Source: CAD feature listing. Evaluate the final solid. Frame: model axes, mm. Face numbers are marked on the shaded views. A direction names the side the tool comes from. Round coordinates to 2 decimals unless told otherwise and drop trailing zeros. Order: outer loops, then holes, each group sorted by start corner. A loop starts at its lowest first (then second) coordinate and runs counter-clockwise, first axis right, second up. Notation, with made-up numbers: (64.5, 28) - (84.5, 28) arc R20 ccw to (84.5, 32) - close; hole circle Ø11 at (18, 68.5). An arc over 180 degrees is marked (long way). Return JSON: item names as keys, results as strings. Group by question number.
1) Contact query for flat-ended pins moving along their axis: P1, Ø4, axis at y = -20, z = 15.5, coming from the -X side; P2, Ø4, axis at x = -21.5, y = -4.5, coming from the -Z side; P3, Ø3, axis at x = -20.5, y = -11.5, coming from the +Z side; P4, Ø10, axis at y = -18.5, z = -10, coming from the +X side. Output: stop coordinate, or through.
2) Section D-D, the plane y = -6.5. Return loops of the section in (x, z), plus the area to 3 significant figures.
3) Ray query, line 1 (X direction, y = -15.75, z = 2); line 2 (X direction, y = -6.75, z = -2); line 3 (Z direction, x = 13.5, y = -12.5). Return the intervals inside material, ascending. Write a range as from..to.
4) Section B-B, the plane x = 23.5. Return loops of the section in (y, z).
5) Access query for the marked faces 1, 2 and 3. Directions: +Z, -Z, +X, -X, +Y, -Y. A direction counts if a zero-diameter tool reaches every point of the face in a straight line with its end or side. Return the directions, or none.
6) Mould query, pull axis Z, two halves, no side actions, for the marked faces 4, 5, 6 and 7. Classes: pulls with the +Z half, pulls with the -Z half, needs draft (parallel to the pull), parting line crosses it, or undercut.
7) Section C-C, the plane y = -16.5. Return loops of the section in (x, z).
8) Section A-A, the plane z = -23.5. Return loops of the section in (x, y), plus the area to 3 significant figures.
```python
from build123d import *

# Parameters (mm, degrees)
F1_DEPTH = 25.4
F2_R     = 8.4230292531
F3_DEPTH = 15.24
F4_R     = 8.4646694798
F5_DEPTH = 15.24


with BuildPart() as f1:
    # F0 (on Front) → F1 (new body)
    with BuildSketch(Plane.XZ):
        Polygon((0, 51.8097877502), (-6.8899182792, 21.4846514834), (-38.7902185321, 21.4846514834), (-14.4291445613, 0), (-23.4517641366, -28.4915324301), (0, -12.2508164495), (27.0749107003, -28.4915324301), (18.9545508474, 0), (43.3156266809, 21.4846514834), (12.6387169585, 21.4846514834), align=None)
    extrude(amount=F1_DEPTH)

    # F2 (on face) → F3 (cut)
    with BuildSketch(Plane(origin=(-5.4041094275, 0, -9.0091951821), x_dir=(0.8575520342, 0, -0.5143972285), z_dir=(-0.5143972285, 0, -0.8575520342))):
        with Locations((6.3017860283, 12.7)):
            Circle(F2_R)
    extrude(amount=-F3_DEPTH, mode=Mode.SUBTRACT)

    # F4 (on face) → F5 (cut)
    with BuildSketch(Plane(origin=(5.7339883167, 0, -8.279939242), x_dir=(0.8221121344, 0, 0.5693255996), z_dir=(0.5693255996, 0, -0.8221121344))):
        with Locations((-6.9747034212, 12.7)):
            Circle(F4_R)
    extrude(amount=-F5_DEPTH, mode=Mode.SUBTRACT)


solid = f1.part
```
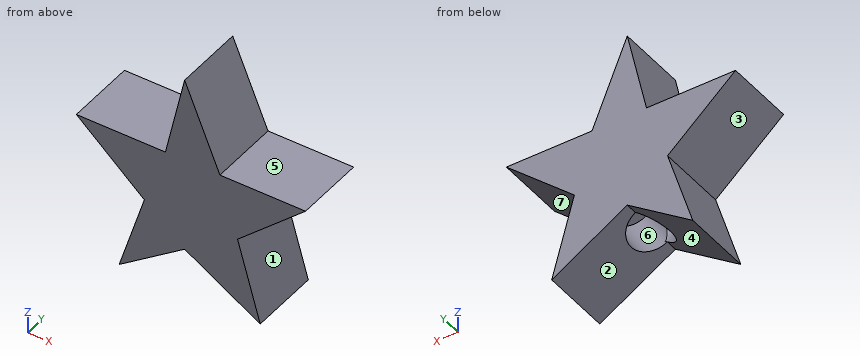
Geometry check:
{
 "1": {"P1": "x = -34.27", "P2": "z = -28.49", "P3": "z = 21.48", "P4": "x = 23.23"},
 "2": {"outline": "(-38.79, 21.48) - (-14.43, 0) - (-23.45, -28.49) - (-4.74, -15.53) - (-13.41, -3) - (-3.94, 3.56) - (-0.31, -1.68) - (2.95, 3.75) - (12.73, -2.11) - (4.89, -15.18) - (27.07, -28.49) - (18.95, 0) - (43.32, 21.48) - (12.64, 21.48) - (0, 51.81) - (-6.89, 21.48) - close", "area": "2,020 mm2"},
 "3": {"line 1": "-16.7..-6.19, 5.87..21.22", "line 2": "-15.06..-11.97, 12.54..19.52", "line 3": "-20.35..-6.11, -2.58..21.48"},
 "4": {"outline": "(-25.4, -26.35) - (0, -26.35) - (0, -15.95) - (-25.4, -15.95) - close; (-25.4, 4.01) - (0, 4.01) - (0, 21.48) - (-25.4, 21.48) - close"},
 "5": {"face 1": "+X, +Y, -Y", "face 2": "-Z, +Y, -Y", "face 3": "-X, +Y, -Y"},
 "6": {"face 4": "pulls with the -Z half", "face 5": "pulls with the +Z half", "face 6": "undercut", "face 7": "undercut"},
 "7": {"outline": "(-38.79, 21.48) - (-14.43, 0) - (-23.45, -28.49) - (-6.22, -16.56) - (-14.89, -4.03) - (-2.46, 4.58) - (-0.43, 1.65) - (1.39, 4.69) - (14.29, -3.05) - (6.45, -16.12) - (27.07, -28.49) - (18.95, 0) - (43.32, 21.48) - (12.64, 21.48) - (0, 51.81) - (-6.89, 21.48) - close"},
 "8": {"outline": "(-21.87, -25.4) - (-16.24, -25.4) - (-16.24, 0) - (-21.87, 0) - close; (18.75, -25.4) - (25.65, -25.4) - (25.65, 0) - (18.75, 0) - close", "area": "318 mm2"}
}
